Can you work these out from the drawing? Everything is in mm from the part's minimum corner. Coordinates: 2 decimals unless noted, no trailing zeros. Order: outer loops, then holes, each group sorted by start corner. A loop starts at its lowest first (then second) coordinate and runs counter-clockwise, first axis right, second up. Notation, with made-up numbers: (68, -28.5) -> (94, -28.5) arc R23 ccw to (94, 6.5) -> close; hole circle Ø9 at (54, 8.25). An arc over 180 degrees is marked (long way). Return JSON: item names as keys, results as strings. Group by question number.
1) If we section it at B-B, the plane x = 33: Please give me the cut outline in (y, z).
2) If we section it at D-D, the plane z = 3.9: Please give me the cut outline in (x, y).
3) If I drill on probe 1 along Z at (x, y) = (4.5, 0.75); probe 2 along X at (y, z) = (1.4, 1.7) (1 decimal); probe 3 along X at (y, z) = (1.5, 1.2) (1 decimal), over which ranges is the centre line in solid material (lowest first)? Write a range as from..to.
4) If we section it at C-C, the plane y = 1.4: Please give me the cut outline in (x, z) (1 decimal), then the cut area to 3 significant figures.
5) If we section it at A-A, the plane z = 2.25: Please give me the cut outline in (x, y) (1 decimal).
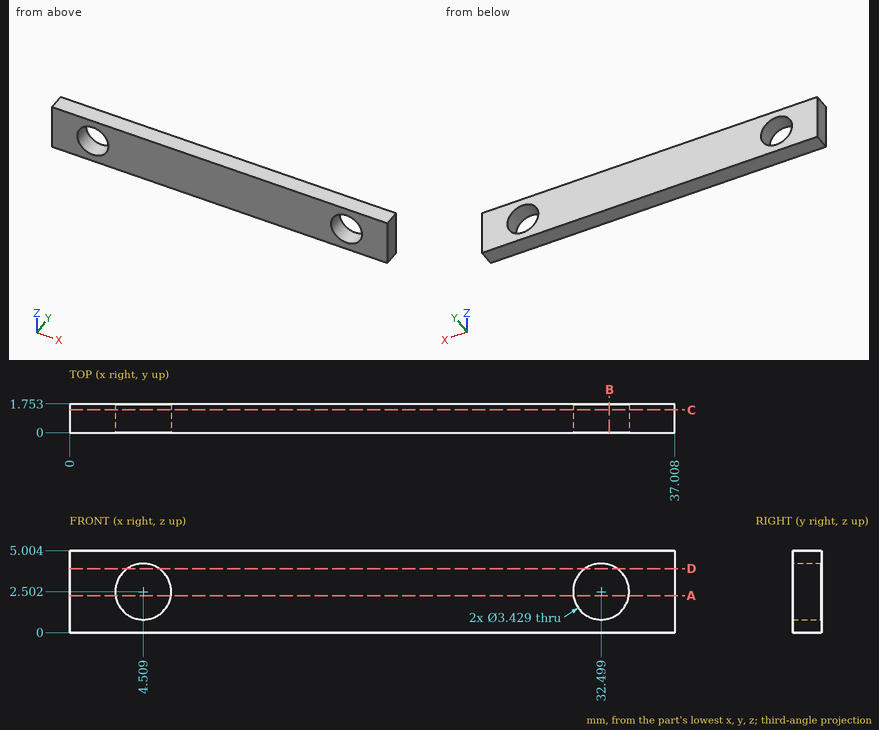
Result sheet:
{
 "1": {"outline": "(0, 0) -> (1.75, 0) -> (1.75, 0.86) -> (0, 0.86) -> close; (0, 4.14) -> (1.75, 4.14) -> (1.75, 5) -> (0, 5) -> close"},
 "2": {"outline": "(0, 0) -> (3.52, 0) -> (3.52, 1.75) -> (0, 1.75) -> close; (5.5, 0) -> (31.51, 0) -> (31.51, 1.75) -> (5.5, 1.75) -> close; (33.49, 0) -> (37.01, 0) -> (37.01, 1.75) -> (33.49, 1.75) -> close"},
 "3": {"probe 1": "z = 0..0.79, 4.22..5", "probe 2": "x = 0..3, 6..31, 34..37", "probe 3": "x = 0..3.4, 5.6..31.4, 33.6..37"},
 "4": {"outline": "(0, 0) -> (37, 0) -> (37, 5) -> (0, 5) -> close; hole circle Ø3.4 at (4.5, 2.5); hole circle Ø3.4 at (32.5, 2.5)", "area": "167 mm2"},
 "5": {"outline": "(0, 0) -> (2.8, 0) -> (2.8, 1.8) -> (0, 1.8) -> close; (6.2, 0) -> (30.8, 0) -> (30.8, 1.8) -> (6.2, 1.8) -> close; (34.2, 0) -> (37, 0) -> (37, 1.8) -> (34.2, 1.8) -> close"}
}
